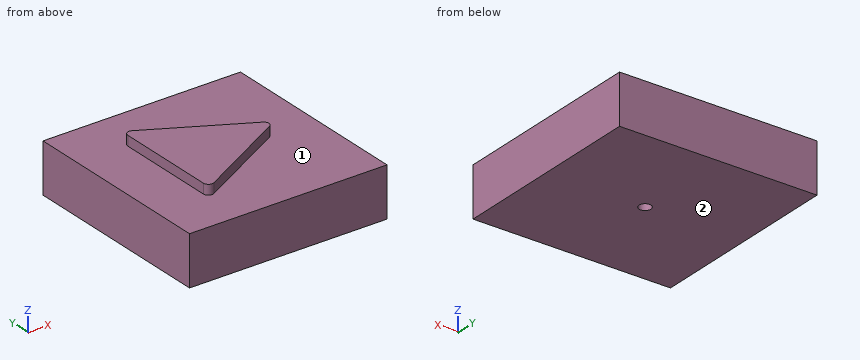
```python
from build123d import *

# Parameters (mm, degrees)
SKETCH1_W           = 20
SKETCH1_H           = 20
BOSS_EXTRUDE1_DEPTH = 5
SKETCH6_R           = 0.6
CUT_EXTRUDE1_DEPTH  = 5
BOSS_EXTRUDE2_DEPTH = 1


with BuildPart() as part:
    # Sketch1 → Boss-Extrude1 (new body)
    with BuildSketch(Plane.XY):
        Rectangle(SKETCH1_W, SKETCH1_H)
    extrude(amount=BOSS_EXTRUDE1_DEPTH)

    # Sketch6 → Cut-Extrude1 (cut)
    with BuildSketch(Plane.XY.offset(5)):
        Circle(SKETCH6_R)
    extrude(amount=-CUT_EXTRUDE1_DEPTH, mode=Mode.SUBTRACT)

    # Sketch2 → Boss-Extrude2 (add)
    with BuildSketch(Plane.XY.offset(5)):
        with BuildLine():
            Line((-5, 5.157728905), (-5, -5.157728905))
            ThreePointArc((-5, -5.157728905), (-4.755232215, -5.58767834), (-4.260573935, -5.596676692))
            Line((-4.260573935, -5.596676692), (5.195262391, -0.438947786))
            ThreePointArc((5.195262391, -0.438947786), (5.455836326, 0), (5.195262391, 0.438947786))
            Line((5.195262391, 0.438947786), (-4.260573935, 5.596676692))
            ThreePointArc((-4.260573935, 5.596676692), (-4.755232215, 5.58767834), (-5, 5.157728905))
        make_face()
    extrude(amount=BOSS_EXTRUDE2_DEPTH)


solid = part.part
```
Design review of the part built by this model. Coordinates are the model's own, in mm. Face numbers are marked on the shaded views. A direction names the side the tool comes from. Give positions to 0.01 mm unless a question says otherwise; leave off trailing zeros. Order: outer loops, then holes, each group sorted by start corner. A loop starts at its lowest first (then second) coordinate and runs counter-clockwise, first axis right, second up. Notation, with made-up numbers: (-7, 17.5) - (35, 17.5) arc R35 cw to (35, 50.5) - close; hole circle Ø4 at (-27.5, 10.25). An arc over 180 degrees is marked (long way). Use a Markdown table: item, result. Add a question column.
(1) Clearance check with flat-ended pins moving along their axes: P1, Ø2, axis at x = 5, y = -1, coming from the -Z side; P2, Ø0.8, axis at y = 2.5, z = 5.5, coming from the -X side. State where each tip first meets the part, or that it passes through.
(2) Machinability: for the marked faces 1 and 2, which of the approach directions +Z, -Z, +X, -X, +Y, -Y give a long, thin tool a straight path to every point of the face, cutting with its end or side? Answer none if there is none.
(3) Wall thickness on probe 1 along Y at (x, z) = (0, 3.55); probe 2 along Z at (x, y) = (-8.5, -0.75); probe 3 along Y at (x, z) = (-0.25, 3.2): over which ranges is each line inside the solid? List them lowest first. Write a range as [from, to].
(4) Add section B-B on z = 5.3. Give the boundary of the cut face in (x, y), then the cut area to 3 significant figures.
(5) Add section A-A on y = 0. Give the boundary of the cut face in (x, z).
(6) Add section D-D on x = 8.5. Give the boundary of the cut face in (y, z).
(7) Add section C-C on x = 0. Give the boundary of the cut face in (y, z).
Report:
| question | item | result |
|---|---|---|
| 1 | P1 | stops at z = 0 |
| 1 | P2 | stops at x = -5 |
| 2 | face 1 | +Z |
| 2 | face 2 | -Z, +X, -X, +Y, -Y |
| 3 | probe 1 | y = [-10, -0.6], [0.6, 10] |
| 3 | probe 2 | z = [0, 5] |
| 3 | probe 3 | y = [-10, -0.55], [0.55, 10] |
| 4 | outline | (-5, -5.16) arc R0.5 ccw to (-4.26, -5.6) - (5.2, -0.44) arc R0.5 ccw to (5.2, 0.44) - (-4.26, 5.6) arc R0.5 ccw to (-5, 5.16) - close |
| 4 | area | 65.5 mm² |
| 5 | outline | (-10, 0) - (-0.6, 0) - (-0.6, 5) - (0.6, 5) - (0.6, 0) - (10, 0) - (10, 5) - (5.46, 5) - (5.46, 6) - (-5, 6) - (-5, 5) - (-10, 5) - close |
| 6 | outline | (-10, 0) - (10, 0) - (10, 5) - (-10, 5) - close |
| 7 | outline | (-10, 0) - (-0.6, 0) - (-0.6, 5) - (0.6, 5) - (0.6, 0) - (10, 0) - (10, 5) - (3.27, 5) - (3.27, 6) - (-3.27, 6) - (-3.27, 5) - (-10, 5) - close |
